```python
from build123d import *

# Parameters (mm, degrees)
F0_R     = 8.5
F1_DEPTH = 6


with BuildPart() as f1:
    # F0 (on Top) → F1 (new body)
    with BuildSketch(Plane.XY):
        with BuildLine():
            ThreePointArc((8.182061, 17.918919), (10.638226, 21.632146), (11.5, 26))
            ThreePointArc((11.5, 26), (-4.367854, 36.638226), (-8.182061, 17.918919))
            ThreePointArc((-8.182061, 17.918919), (0, 14.5), (8.182061, 17.918919))
        make_face()
        with Locations((0, 26)):
            Circle(F0_R, mode=Mode.SUBTRACT)
        with BuildLine():
            ThreePointArc((8.182061, 17.918919), (0, 14.5), (-8.182061, 17.918919))
            ThreePointArc((-8.182061, 17.918919), (-6.162447, 13), (-8.182061, 8.081081))
            ThreePointArc((-8.182061, 8.081081), (0, 11.5), (8.182061, 8.081081))
            ThreePointArc((8.182061, 8.081081), (6.162447, 13), (8.182061, 17.918919))
        make_face()
        with BuildLine():
            ThreePointArc((8.182061, 8.081081), (0, 11.5), (-8.182061, 8.081081))
            ThreePointArc((-8.182061, 8.081081), (-9.959292, 5.75), (-11.089452, 3.045332))
            ThreePointArc((-11.089452, 3.045332), (-9.959292, -5.75), (-2.907391, -11.126414))
            ThreePointArc((-2.907391, -11.126414), (0, -11.5), (2.907391, -11.126414))
            ThreePointArc((2.907391, -11.126414), (9.101785, -7.029047), (11.5, 0))
            ThreePointArc((11.5, 0), (11.396901, 1.536441), (11.089452, 3.045332))
            ThreePointArc((11.089452, 3.045332), (9.959292, 5.75), (8.182061, 8.081081))
        make_face()
        Circle(F0_R, mode=Mode.SUBTRACT)
        with BuildLine():
            ThreePointArc((-2.907391, -11.126414), (-9.959292, -5.75), (-11.089452, 3.045332))
            ThreePointArc((-11.089452, 3.045332), (-14.339554, -1.163165), (-19.60927, -1.873586))
            ThreePointArc((-19.60927, -1.873586), (-13.414875, -5.970953), (-11.01666, -13))
            ThreePointArc((-11.01666, -13), (-11.11976, -14.536441), (-11.427208, -16.045332))
            ThreePointArc((-11.427208, -16.045332), (-8.177107, -11.836835), (-2.907391, -11.126414))
        make_face()
        with BuildLine():
            ThreePointArc((-11.01666, -13), (-13.414875, -5.970953), (-19.60927, -1.873586))
            ThreePointArc((-19.60927, -1.873586), (-32.475953, -18.75), (-11.427208, -16.045332))
            ThreePointArc((-11.427208, -16.045332), (-11.11976, -14.536441), (-11.01666, -13))
        make_face()
        with Locations((-22.51666, -13)):
            Circle(F0_R, mode=Mode.SUBTRACT)
        with BuildLine():
            ThreePointArc((19.60927, -1.873586), (14.339554, -1.163165), (11.089452, 3.045332))
            ThreePointArc((11.089452, 3.045332), (11.396901, 1.536441), (11.5, 0))
            ThreePointArc((11.5, 0), (9.101785, -7.029047), (2.907391, -11.126414))
            ThreePointArc((2.907391, -11.126414), (8.177107, -11.836835), (11.427208, -16.045332))
            ThreePointArc((11.427208, -16.045332), (12.557368, -7.25), (19.60927, -1.873586))
        make_face()
        with BuildLine():
            ThreePointArc((34.01666, -13), (29.545708, -3.898215), (19.60927, -1.873586))
            ThreePointArc((19.60927, -1.873586), (12.557368, -7.25), (11.427208, -16.045332))
            ThreePointArc((11.427208, -16.045332), (24.053101, -24.396901), (34.01666, -13))
        make_face()
        with Locations((22.51666, -13)):
            Circle(F0_R, mode=Mode.SUBTRACT)
    extrude(amount=F1_DEPTH)


solid = f1.part
```
The listing builds one solid part. Answer for the finished solid, in the listing's coordinates (mm). A direction names the side the tool comes from. Coordinates: 2 decimals unless noted, no trailing zeros. Write each loop counter-clockwise with the first axis right and the second up, starting at its lowest first coordinate (ties: lowest second). Pieces come first, ordered by that corner, then holes. Notation, with made-up numbers: (87, -10) -> (126, -10) arc R19 cw to (126, 1) -> close; hole circle Ø8 at (-29, 38.25). An arc over 180 degrees is marked (long way). Write each question's results on one line, items separated by ' | '. Start each with the question number.
1) A cutting plane is placed at B-B (y = 0). Determine the outline of the cut face in (x, z).
2) Straight lines are drawn through the part: probe 1 along Y at (x, z) = (23, 5); probe 2 along X at (y, z) = (-6, 2.4); probe 3 along X at (y, z) = (-15, 2.05). For each, find the intervals that lie inside material, in ascending order.
3) For a pull along Y with two mould halves and no side action, classify faces 4 (the cylindrical face through (-6.163, 13.076, 2.958)), 5 (the cylindrical face through (-8.243, -11.875, 2.958)), 6 (the flat face through (0, 9, 6)) as +Y half, -Y half, draft (parallel to the pull), parting line (faces both ways), or undercut.
4) Flat-ended cylindrical pins translate along their axes: pin 1 Ø1.5 at (x, z) = (16.5, 2.5) entering from +Y; pin 2 Ø3 at (y, z) = (-4.5, 1) entering from -X; pin 3 Ø2 at (y, z) = (22, 1) entering from -X; pin 4 Ø22 at (x, y) = (22.52, -13) entering from -Z. Find the tip coordinate at first contact, or state that the pin passes through.
5) A cutting plane is placed at D-D (z = 1.45). Determine the outline of the cut face in (x, y), then the cut area to 3 significant figures.
6) A cutting plane is placed at C-C (x = -24.5). Determine the outline of the cut face in (y, z), then the cut area to 3 significant figures.
7) A tool of negligible diameter and unlimited length cuts with its end or side. For faces 1 (the cylindrical face through (4.57, 7.167, 2.958)), 2 (the cylindrical face through (9.98, 5.71, 2.96)), 3 (the cylindrical face through (-9.939, 5.786, 2.958)), from which of +Z, -Z, +X, -X, +Y, -Y can it reach the whole face along a straight path? Write none if from no direction.
8) A cutting plane is placed at A-A (x = 0). Determine the outline of the cut face in (y, z), then the cut area to 3 significant figures.
Values follow:
1) outline: (-12.84, 0) -> (-8.5, 0) -> (-8.5, 6) -> (-12.84, 6) -> close; (8.5, 0) -> (12.84, 0) -> (12.84, 6) -> (8.5, 6) -> close
2) probe 1: -24.49 to -21.49, -4.51 to -1.51 | probe 2: -31.64 to -27.34, -17.69 to -6.02, 6.02 to 17.69, 27.34 to 31.64 | probe 3: -33.84 to -30.78, -14.26 to -11.05, 11.05 to 14.26, 30.78 to 33.84
3) face 4: undercut | face 5: -Y half | face 6: draft
4) pin 1: y = -1.78 | pin 2: x = -31.64 | pin 3: x = -11.1 | pin 4: z = 0
5) outline: (-19.61, -1.87) arc R11.5 ccw (long way) to (-11.43, -16.05) arc R7 cw to (-2.91, -11.13) arc R11.5 ccw to (2.91, -11.13) arc R7 cw to (11.43, -16.05) arc R11.5 ccw (long way) to (19.61, -1.87) arc R7 cw to (11.09, 3.05) arc R11.5 ccw to (8.18, 8.08) arc R7 cw to (8.18, 17.92) arc R11.5 ccw to (11.5, 26) arc R11.5 ccw (long way) to (-8.18, 17.92) arc R7 cw to (-8.18, 8.08) arc R11.5 ccw to (-11.09, 3.05) arc R7 cw to start; hole circle Ø17 at (-22.52, -13); hole circle Ø17 at (0, 0); hole circle Ø17 at (0, 26); hole circle Ø17 at (22.52, -13) | area: 923 mm²
6) outline: (-24.33, 0) -> (-21.27, 0) -> (-21.27, 6) -> (-24.33, 6) -> close; (-4.73, 0) -> (-1.67, 0) -> (-1.67, 6) -> (-4.73, 6) -> close | area: 36.7 mm²
7) face 1: +Z, -Z | face 2: +Z, -Z, +X | face 3: +Z, -Z, -X
8) outline: (-11.5, 0) -> (-8.5, 0) -> (-8.5, 6) -> (-11.5, 6) -> close; (8.5, 0) -> (17.5, 0) -> (17.5, 6) -> (8.5, 6) -> close; (34.5, 0) -> (37.5, 0) -> (37.5, 6) -> (34.5, 6) -> close | area: 90.0 mm²
